from build123d import *

# Parameters (mm, degrees)
BOSS_EXTRUDE1_DEPTH   = 50.8
BOSS_EXTRUDE1_2_DEPTH = 50.8
SKETCH2_R             = 6.35
BOSS_EXTRUDE2_DEPTH   = 50.8


with BuildPart() as part:
    # Sketch1 → Boss-Extrude1 (new body)
    with BuildSketch(Plane.XY):
        with BuildLine():
            ThreePointArc((-11.952941176, 49.373750083), (0, 50.8), (11.952941176, 49.373750083))
            ThreePointArc((11.952941176, 49.373750083), (15.78585938, 51.712550639), (13.447058824, 55.545468843))
            ThreePointArc((13.447058824, 55.545468843), (0, 57.15), (-13.447058824, 55.545468843))
            ThreePointArc((-13.447058824, 55.545468843), (-15.78585938, 51.712550639), (-11.952941176, 49.373750083))
        make_face()
    extrude(amount=-BOSS_EXTRUDE1_DEPTH)



with BuildPart() as body_2:
    # Sketch1 → Boss-Extrude1 2 (new body)
    with BuildSketch(Plane.XY):
        with BuildLine():
            ThreePointArc((-10.586266882, 46.303249967), (0, 47.498), (10.586266882, 46.303249967))
            ThreePointArc((10.586266882, 46.303249967), (12.973765752, 42.500474776), (9.170990561, 40.112975907))
            ThreePointArc((9.170990561, 40.112975907), (0, 41.148), (-9.170990561, 40.112975907))
            ThreePointArc((-9.170990561, 40.112975907), (-12.973765752, 42.500474776), (-10.586266882, 46.303249967))
        make_face()
    extrude(amount=-BOSS_EXTRUDE1_2_DEPTH)


with BuildPart() as part_1:
    add(part.part)

    add(body_2.part)  # Boss-Extrude2 merges body 2
    # Sketch2 → Boss-Extrude2 (add)
    with BuildSketch(Plane.XY):
        with Locations(Location((0, 49.149, 0), (0, 0, 168.476640001))):
            Circle(SKETCH2_R)
    extrude(amount=BOSS_EXTRUDE2_DEPTH)


solid = part_1.part
Read the model definition and answer for the solid it produces. Units are mm, in the model's axes. A direction names the side the tool comes from. Round coordinates to 2 decimals unless told otherwise and drop trailing zeros. Write each loop counter-clockwise with the first axis right and the second up, starting at its lowest first coordinate (ties: lowest second). Pieces come first, ordered by that corner, then holes.
1. Given pin 1 Ø2 at (x, z) = (2, 27.5) entering from -Y; pin 2 Ø6 at (y, z) = (43, -21.5) entering from +X; pin 3 Ø5 at (y, z) = (46, -14.5) entering from -X, each flat-ended and moving along its own axis, determine where each tip first touches the part or whether it passes through.
2. The part is cut by section D-D, the plane x = -4.5. Determine the outline of the cut face in (y, z).
3. The part is cut by section C-C, the plane y = 53. Determine the outline of the cut face in (x, z), then the cut area to 3 significant figures.
4. Determine the mould class of faces 1 (the face through (0, 53, -50.8)), 2 (the face through (-0.2, 50.8, -25)), 3 (the face through (3.73, 44.01, 25.04)), 4 (the face through (12.99, 42.57, -25.04)) for opening direction Y: pulls with the +Y half, pulls with the -Y half, needs draft (parallel to the pull), parting line crosses it, or undercut.
5. Straight lines are drawn through the part: L1, parallel to Z at x = -11, y = 55.75; L2, parallel to X at y = 43, z = -38.5; L3, parallel to Y at x = 11.5, z = -24. For each, find the intervals that lie inside material, in ascending order.
6. Which of the six approach directions +Z, -Z, +X, -X, +Y, -Y give full straight-line access (tool end or side, diameter ignored) to faces 5 (the face through (0, 49, 0)), 6 (the face through (0.129, 41.148, -25.044)), 7 (the face through (0, 56, 0)), 8 (the face through (0, 42, 0)), 9 (the face through (0, 44, -50.8))?
7. The part is cut by section A-A, the plane z = -20. Determine the outline of the cut face in (x, y) (3 decimals).
8. The part is cut by section B-B, the plane x = 0. Determine the outline of the cut face in (y, z).
Values:
1. pin 1: stops at y = 42.88
1. pin 2: stops at x = 13.05
1. pin 3: stops at x = -13.04
2. outline: (40.9, -50.8) - (47.28, -50.8) - (47.28, 0) - (50.6, 0) - (50.6, -50.8) - (56.97, -50.8) - (56.97, 0) - (53.63, 0) - (53.63, 50.8) - (44.67, 50.8) - (44.67, 0) - (40.9, 0) - close
3. outline: (-15.83, -50.8) - (15.83, -50.8) - (15.83, 0) - (5.05, 0) - (5.05, 50.8) - (-5.05, 50.8) - (-5.05, 0) - (-15.83, 0) - close
3. area: 2,120 mm2
4. face 1: needs draft
4. face 2: undercut
4. face 3: parting line crosses it
4. face 4: undercut
5. L1: z = -50.8 to 0
5. L2: x = -13.05 to 13.05
5. L3: y = 40.48 to 45.94, 49.48 to 55.98
6. face 5: -Z
6. face 6: +Z, -Z, -Y
6. face 7: +Z, +Y
6. face 8: +Z, -Y
6. face 9: -Z, +X, -X, +Y, -Y
7. outline: (-13.447, 55.545) arc R3.175 ccw to (-11.953, 49.374) arc R50.8 cw to (11.953, 49.374) arc R3.175 ccw to (13.447, 55.545) arc R57.15 ccw to start; (-10.586, 46.303) arc R3.175 ccw to (-9.171, 40.113) arc R41.148 cw to (9.171, 40.113) arc R3.175 ccw to (10.586, 46.303) arc R47.498 ccw to start
8. outline: (41.15, -50.8) - (47.5, -50.8) - (47.5, 0) - (50.8, 0) - (50.8, -50.8) - (57.15, -50.8) - (57.15, 0) - (55.5, 0) - (55.5, 50.8) - (42.8, 50.8) - (42.8, 0) - (41.15, 0) - close
